Geometry check sheet. Reference: the model listing, model coordinates, mm. A direction names the side the tool comes from. Round coordinates to 2 decimals unless told otherwise and drop trailing zeros. Loops run counter-clockwise (first coordinate to the right, second up) from the corner with the lowest first, then second, coordinate; pieces in that order, holes last. Notation, with made-up numbers: (-33.75, 25) - (-27.75, 25) arc R18 cw to (-27.75, 48) - close; hole circle Ø5 at (-10.75, -5.5). An arc over 180 degrees is marked (long way). Answer in a Markdown table with one row per item. Add a question column.
```python
from build123d import *

# Parameters (mm, degrees)
BOX_W             = 141
BOX_H             = 73.6
BOX_DEPTH         = 22.5
FILLET_R          = 3
CYLINDER002_R     = 1.8
CYLINDER002_DEPTH = 10
BOX006_W          = 10
BOX006_H          = 78.6
BOX006_DEPTH      = 25
FILLET007_R       = 4
CYLINDER001_R     = 2.1
CYLINDER001_DEPTH = 10
BOX003_W          = 10
BOX003_H          = 10
BOX003_DEPTH      = 9
FILLET003_R       = 3
BOX007_W          = 10
BOX007_H          = 100
BOX007_DEPTH      = 3
FILLET006_R       = 3


with BuildPart() as battery_fillet:
    # Box → Box (new body)
    with BuildSketch(Plane(origin=(2, 0, 0), x_dir=(1, 0, 0), z_dir=(0, 0, 1))):
        with Locations((70.5, 36.8)):
            Rectangle(BOX_W, BOX_H)
    extrude(amount=BOX_DEPTH)

    # Fillet
    fillet_edges = [battery_fillet.edges().sort_by_distance(p)[0] for p in [
        (72.5, 0, 0),
        (72.5, 0, 22.5),
        (72.5, 73.6, 0),
        (72.5, 73.6, 22.5),
    ]]
    fillet(fillet_edges, radius=FILLET_R)


with BuildPart() as battery_fillet_1:
    # Fillet placement: moved
    add(battery_fillet.part.moved(Location((0, -36.8, 0))))


with BuildPart() as bolt_hole001:
    # Cylinder002 → Cylinder002 (new body)
    with BuildSketch(Plane(origin=(5, 45, 0), x_dir=(1, 0, 0), z_dir=(0, 0, 1))):
        Circle(CYLINDER002_R)
    extrude(amount=CYLINDER002_DEPTH)


with BuildPart() as bolt_hole_fusion001:
    # Part__Mirroring002: instance of bolt hole001
    add(bolt_hole001.part.mirror(Plane(origin=(0, 0, 0), x_dir=(1, 0, 0), z_dir=(0, 1, 0))))

    # Fusion002: union bolt hole001
    add(bolt_hole001.part)


with BuildPart() as back_wall_fillet001:
    # Box006 → Box006 (new body)
    with BuildSketch(Plane(origin=(0, -39.3, 0), x_dir=(1, 0, 0), z_dir=(0, 0, 1))):
        with Locations((5, 39.3)):
            Rectangle(BOX006_W, BOX006_H)
    extrude(amount=BOX006_DEPTH)

    # Fillet007
    fillet007_edges = [back_wall_fillet001.edges().sort_by_distance(p)[0] for p in [
        (5, -39.3, 25),
        (5, 39.3, 25),
    ]]
    fillet(fillet007_edges, radius=FILLET007_R)


with BuildPart() as insert_hole:
    # Cylinder001 → Cylinder001 (new body)
    with BuildSketch(Plane(origin=(5, 0, 0), x_dir=(1, 0, 0), z_dir=(0, 0, 1))):
        Circle(CYLINDER001_R)
    extrude(amount=CYLINDER001_DEPTH)


with BuildPart() as top_insert_box_cut:
    # Box003 → Box003 (new body)
    with BuildSketch(Plane(origin=(0, -5, 0), x_dir=(1, 0, 0), z_dir=(0, 0, 1))):
        with Locations((5, 5)):
            Rectangle(BOX003_W, BOX003_H)
    extrude(amount=BOX003_DEPTH)

    # Fillet003
    fillet003_edges = [top_insert_box_cut.edges().sort_by_distance(p)[0] for p in [
        (0, -5, 4.5),
        (0, 5, 4.5),
        (10, -5, 4.5),
        (10, 5, 4.5),
    ]]
    fillet(fillet003_edges, radius=FILLET003_R)

    # Cut: cut insert hole
    add(insert_hole.part, mode=Mode.SUBTRACT)


with BuildPart() as top_insert_box_cut_1:
    # Cut placement: moved
    add(top_insert_box_cut.part.moved(Location((0, 30, 25))))


with BuildPart() as part_mirroring001:
    # Part__Mirroring001: instance of top insert box cut
    add(top_insert_box_cut_1.part.mirror(Plane(origin=(0, 0, 0), x_dir=(1, 0, 0), z_dir=(0, 1, 0))))


with BuildPart() as battery_frame:
    # Box007 → Box007 (new body)
    with BuildSketch(Plane(origin=(0, -50, 0), x_dir=(1, 0, 0), z_dir=(0, 0, 1))):
        with Locations((5, 50)):
            Rectangle(BOX007_W, BOX007_H)
    extrude(amount=BOX007_DEPTH)

    # Fillet006
    fillet006_edges = [battery_frame.edges().sort_by_distance(p)[0] for p in [
        (0, -50, 1.5),
        (0, 50, 1.5),
        (10, -50, 1.5),
        (10, 50, 1.5),
    ]]
    fillet(fillet006_edges, radius=FILLET006_R)

    # Fusion003: union back wall fillet001, top insert box cut, Part__Mirroring001
    add(back_wall_fillet001.part)
    add(top_insert_box_cut_1.part)
    add(part_mirroring001.part)

    # Cut005: cut bolt hole fusion001
    add(bolt_hole_fusion001.part, mode=Mode.SUBTRACT)


with BuildPart() as battery_frame_1:
    # Cut005 placement: moved
    add(battery_frame.part.moved(Location((100, 0, 0))))

    # Cut006: cut battery fillet
    add(battery_fillet_1.part, mode=Mode.SUBTRACT)


solid = battery_frame_1.part
```
Q1. Cross-section at D-D, the plane x = 101.5. Enter the section's corners in (y, z).
Q2. Release check for a two-part mould opening along Y. For faces 5 (the cylindrical face through (109.14, -34.1, 29.56)), 6 (the cylindrical face through (100.86, 49.1, 1.52)), 7 (the cylindrical face through (102.9, 30.09, 29.44)) record: +Y half, -Y half, draft (parallel to the pull), parting line (faces both ways), or undercut.
Q3. Cross-section at C-C, the plane y = -30. Enter the section's corners in (x, z), plus the area to 3 significant figures.
Q4. Set-up check for faces 1 (the cylindrical face through (100.86, -34.1, 29.56)), 2 (the cylindrical face through (100.86, 25.9, 29.56)), 3 (the cylindrical face through (109.14, 34.1, 29.56)), 4 (the flat face through (105, 30, 25)): record each of +Z, -Z, +X, -X, +Y, -Y from which the full face is reachable in a straight line by a thin tool's end or side.
Q5. Cross-section at A-A, the plane y = 45. Enter the section's corners in (x, z).
Q6. Depth check by flat-ended pin: P1, Ø2, axis at x = 106, z = 29, coming from the -Y side; P2, Ø1, axis at x = 102, z = 4.5, coming from the +Y side; P3, Ø2, axis at x = 105, y = 45, coming from the +Z side; P4, Ø1.5, axis at x = 109, y = 6.5, coming from the +Z side. Enter the tip coordinate at first touch or a pass-through.
Q7. Scan lines: line 1 (Y direction, x = 105, z = 30.5); line 2 (Y direction, x = 100.5, z = 11); line 3 (X direction, y = -30, z = 31). Record each from-to range of solid material in increasing order. Write a range as from..to.
Q8. Cross-section at B-B, the plane z = 14.5. Enter the section's corners in (x, y), plus the area to 3 significant figures.
Check sheet entries:
| question | item | result |
|---|---|---|
| 1 | outline | (-49.6, 0) - (-33.8, 0) arc R3 cw to (-36.8, 3) - (-36.8, 19.5) arc R3 cw to (-33.8, 22.5) - (33.8, 22.5) arc R3 cw to (36.8, 19.5) - (36.8, 3) arc R3 cw to (33.8, 0) - (49.6, 0) - (49.6, 3) - (39.3, 3) - (39.3, 21) arc R4 ccw to (35.3, 25) - (34.6, 25) - (34.6, 34) - (25.4, 34) - (25.4, 25) - (-25.4, 25) - (-25.4, 34) - (-34.6, 34) - (-34.6, 25) - (-35.3, 25) arc R4 ccw to (-39.3, 21) - (-39.3, 3) - (-49.6, 3) - close |
| 2 | face 5 | -Y half |
| 2 | face 6 | +Y half |
| 2 | face 7 | undercut |
| 3 | outline | (100, 22.5) - (110, 22.5) - (110, 34) - (107.1, 34) - (107.1, 25) - (102.9, 25) - (102.9, 34) - (100, 34) - close |
| 3 | area | 77.2 mm² |
| 4 | face 1 | +Z, -X, -Y |
| 4 | face 2 | +Z, -X |
| 4 | face 3 | +Z, +X, +Y |
| 4 | face 4 | +Z |
| 5 | outline | (100, 0) - (103.2, 0) - (103.2, 3) - (100, 3) - close; (106.8, 0) - (110, 0) - (110, 3) - (106.8, 3) - close |
| 6 | P1 | y = -35 |
| 6 | P2 | y = 39.3 |
| 6 | P3 | through |
| 6 | P4 | z = 25 |
| 7 | line 1 | -35..-32.1, -27.9..-25, 25..27.9, 32.1..35 |
| 7 | line 2 | -39.3..-36.8, 36.8..39.3 |
| 7 | line 3 | 100..102.9, 107.1..110 |
| 8 | outline | (100, -39.3) - (110, -39.3) - (110, -36.8) - (100, -36.8) - close; (100, 36.8) - (110, 36.8) - (110, 39.3) - (100, 39.3) - close |
| 8 | area | 50.0 mm² |
